from build123d import *

# Parameters (mm, degrees)
SKETCH2_W           = 156
SKETCH2_H           = 48
SKETCH2_R           = 2.05
SKETCH2_R_2         = 7.05
BOSS_EXTRUDE2_DEPTH = 3.175
FILLET1_R           = 8


with BuildPart() as part:
    # Sketch2 → Boss-Extrude2 (new body)
    with BuildSketch(Plane.XY):
        Rectangle(SKETCH2_W, SKETCH2_H)
        with Locations((-70, 8)):
            Circle(SKETCH2_R, mode=Mode.SUBTRACT)
        with Locations((-54, 8)):
            Circle(SKETCH2_R, mode=Mode.SUBTRACT)
        with Locations((-54, -8)):
            Circle(SKETCH2_R, mode=Mode.SUBTRACT)
        with Locations((-70, -8)):
            Circle(SKETCH2_R, mode=Mode.SUBTRACT)
        with Locations((47.795580317, 0)):
            Circle(SKETCH2_R_2, mode=Mode.SUBTRACT)
        with Locations((-62, 0)):
            Circle(SKETCH2_R_2, mode=Mode.SUBTRACT)
        with Locations((72, 18)):
            Circle(SKETCH2_R, mode=Mode.SUBTRACT)
        with Locations((72, -18)):
            Circle(SKETCH2_R, mode=Mode.SUBTRACT)
        with Locations((-72, -18)):
            Circle(SKETCH2_R, mode=Mode.SUBTRACT)
        with Locations((-72, 18)):
            Circle(SKETCH2_R, mode=Mode.SUBTRACT)
    extrude(amount=BOSS_EXTRUDE2_DEPTH)

    # Fillet1
    fillet1_edges = [part.edges().sort_by_distance(p)[0] for p in [
        (78, 24, 1.5875),
        (78, -24, 1.5875),
        (-78, -24, 1.5875),
        (-78, 24, 1.5875),
    ]]
    fillet(fillet1_edges, radius=FILLET1_R)


solid = part.part
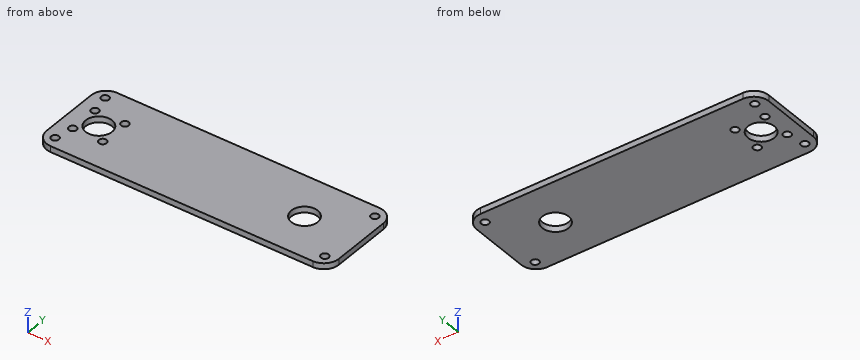
Geometry: final body of the model. Coordinates: model frame, mm. Coordinates: 2 decimals unless noted, no trailing zeros. Loops run counter-clockwise (first coordinate to the right, second up) from the corner with the lowest first, then second, coordinate; pieces in that order, holes last. Notation, with made-up numbers: M -35.5,85.5 L -18.5,85.5 A17 ccw -18.5,89.5 Z; hole C -19,43 d9. An arc over 180 degrees is marked long. One line per item, written item: value. Start each with the question number.
1) Cut plane D-D (y = -2). Return loops of the section in (x, z) (3 decimals), then the cut area to 3 significant figures.
2) Material intervals for L1, parallel to X at y = 1.5, z = 2.75; L2, parallel to Y at x = -71, z = 1; L3, parallel to X at y = 19.5, z = 2.65, sorted ascending. Write a range as from..to.
3) Cut plane C-C (y = 18). Return loops of the section in (x, z) (3 decimals), then the cut area to 3 significant figures.
4) Cut plane A-A (x = -62). Return loops of the section in (y, z) (3 decimals), then the cut area to 3 significant figures.
5) Cut plane B-B (z = 1.3). Count the separate pieces of the cut face and the enclosed holes in it, then the cut area to 3 significant figures.
Evaluation:
1. outline: M -78,0 L -68.76,0 L -68.76,3.175 L -78,3.175 Z; M -55.24,0 L 41.035,0 L 41.035,3.175 L -55.24,3.175 Z; M 54.556,0 L 78,0 L 78,3.175 L 54.556,3.175 Z
1. area: 409 mm^2
2. L1: -78..-68.89, -55.11..40.91, 54.68..78
2. L2: -23.94..-19.79, -16.21..-9.79, -6.21..6.21, 9.79..16.21, 19.79..23.94
2. L3: -77.19..-73.4, -70.6..70.6, 73.4..77.19
3. outline: M -77.746,0 L -74.05,0 L -74.05,3.175 L -77.746,3.175 Z; M -69.95,0 L 69.95,0 L 69.95,3.175 L -69.95,3.175 Z; M 74.05,0 L 77.746,0 L 77.746,3.175 L 74.05,3.175 Z
3. area: 468 mm^2
4. outline: M -24,0 L -7.05,0 L -7.05,3.175 L -24,3.175 Z; M 7.05,0 L 24,0 L 24,3.175 L 7.05,3.175 Z
4. area: 108 mm^2
5. separate pieces: 1
5. enclosed holes: 10
5. area: 7,020 mm^2
